The model under review builds one solid part; all positions refer to its coordinate system, in mm. Face numbers are marked on the shaded views. Coordinates: 2 decimals unless noted, no trailing zeros. Write each loop counter-clockwise with the first axis right and the second up, starting at its lowest first coordinate (ties: lowest second). Pieces come first, ordered by that corner, then holes. Notation, with made-up numbers: M 62.5,76 L 102.5,76 A15 ccw 102.5,103 Z; hole C 7,34 d5. An arc over 180 degrees is marked long. Answer as a JSON object with one key per item and string values.
Autodesk Inventor part; units mm, degrees
ref_plane "YZ Plane" through (0, 0, 0) normal (1, 0, 0) x (0, 1, 0)
ref_plane "XZ Plane" through (0, 0, 0) normal (0, 1, 0) x (-1, 0, 0)
ref_plane "XY Plane" through (0, 0, 0) normal (0, 0, 1) x (1, 0, 0)
sketch "Esboço1" plane through (0, 0, 0) normal (0, 0, 1) x (1, 0, 0)
  line L0 (0, 0) -> (0, 57)
  line L1 (8.2179, 1.5639) -> (9.7832, 1.5639)
  line L2 (9.7832, 1.5639) -> (9.7832, 0)
  line L3 (7.3887, 0.7346) -> (7.3887, 39.3227)
  line L4 (7.3887, 0.7346) -> (7.3887, 0)
  line L5 (7.3887, 0) -> (9.7832, 0)
  line L6 (9.7832, 0) -> (7.3887, 0)
  line L7 (0.8292, 0) -> (0, 0)
  line L8 (0, 42.2247) -> (0, 57)
  line L9 (0, 42.2247) -> (0, 39.7247)
  line L10 (0, 55.3122) -> (0, 52.8122)
  line L11 (8.2179, 49.9102) -> (8.2179, 1.5639)
  line L12 (0, 42.2247) -> (0, 39.3227)
  line L13 (0, 39.3227) -> (7.3887, 39.3227)
  line L14 (0, 52.8122) -> (0, 49.9102)
  line L15 (8.2179, 49.9102) -> (9.7832, 49.9102)
  line L16 (9.7832, 49.9102) -> (9.7832, 51.9102)
  line L17 (9.7832, 51.9102) -> (0, 51.9102)
revolve "Revolução1" add sketch "Esboço1" angle 360 about axis through (0, 0, 0) along (0, 1, 0)
chamfer "Chanfro2" distance 1 angle 45 1 edges at (-9.7832, 0, 0)
chamfer "Chanfro4" distance 1 angle 45 1 edges at (-9.7832, 51.9102, 0)
sketch "Esboço4" plane through (0, 51.9102, 0) normal (0, 1, 0) x (1, 0, 0)
  circle A0 centre (0, 0) radius 8.7832
hole "Furo2" at (0, 51.9102, 0) direction (0, -1, 0) diameter 3 depth 19.499 tip angle 118
properties part number "roda"
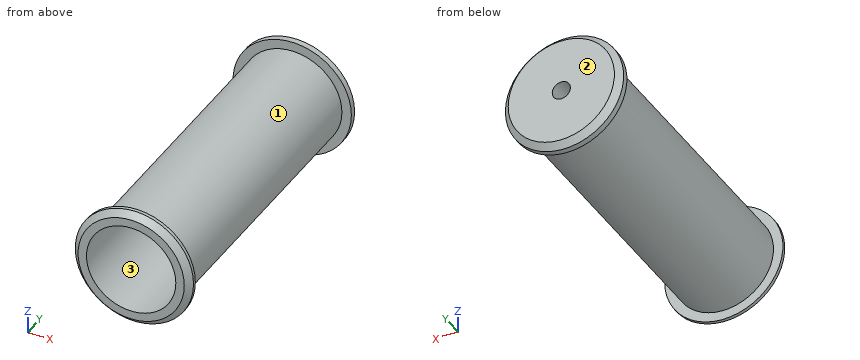
(1) Draft analysis for pull direction Z (two halves, no side actions). For the marked faces 1, 2 and 3, state which applies: released by +Z, released by -Z, zero draft, split by the parting line, or undercut.
Results list:
{"face 1": "split by the parting line", "face 2": "zero draft", "face 3": "undercut"}
(2) Wall thickness on line 1 along Z through (x, y) = (0, 49.75); line 2 along X through (y, z) = (17, 0): over which ranges is each line inside the solid? List them lowest first. Write a range as from..to.
Results list:
{"line 1": "-8.22..-1.5, 1.5..8.22", "line 2": "-8.22..-7.39, 7.39..8.22"}
(3) Add section C-C on y = 15. Give the boundary of the cut face in (x, z).
Results list:
{"outline": "C 0,0 d16.44; hole C 0,0 d14.78"}
(4) Add section D-D on y = 44.5. Give the boundary of the cut face in (x, z), and give its area (3 significant figures).
Results list:
{"outline": "C 0,0 d16.44; hole C 0,0 d3", "area": "205 mm²"}
(5) Add section B-B on z = 0. Give the boundary of the cut face in (x, y).
Results list:
{"outline": "M -9.78,1 L -8.78,0 L -7.39,0 L -7.39,39.32 L -1.5,39.32 L -1.5,51.91 L -8.78,51.91 L -9.78,50.91 L -9.78,49.91 L -8.22,49.91 L -8.22,1.56 L -9.78,1.56 Z; M 1.5,39.32 L 7.39,39.32 L 7.39,0 L 8.78,0 L 9.78,1 L 9.78,1.56 L 8.22,1.56 L 8.22,49.91 L 9.78,49.91 L 9.78,50.91 L 8.78,51.91 L 1.5,51.91 Z"}
(6) Add section A-A on x = 0. Give the boundary of the cut face in (y, z).
Results list:
{"outline": "M 0,-8.78 L 1,-9.78 L 1.56,-9.78 L 1.56,-8.22 L 49.91,-8.22 L 49.91,-9.78 L 50.91,-9.78 L 51.91,-8.78 L 51.91,-1.5 L 39.32,-1.5 L 39.32,-7.39 L 0,-7.39 Z; M 0,7.39 L 39.32,7.39 L 39.32,1.5 L 51.91,1.5 L 51.91,8.78 L 50.91,9.78 L 49.91,9.78 L 49.91,8.22 L 1.56,8.22 L 1.56,9.78 L 1,9.78 L 0,8.78 Z"}
(7) For pin 1 Ø8 at (y, z) = (10.5, 5) entering from +X; pin 2 Ø4.5 at (x, z) = (3.5, 3) entering from -Y; pin 3 Ø1 at (x, y) = (-4.5, 42) entering from -Z, all flat-tipped, find the tip position at first contact; note any pin that passes through.
Results list:
{"pin 1": "x = 8.16", "pin 2": "y = 39.32", "pin 3": "z = -7.18"}
